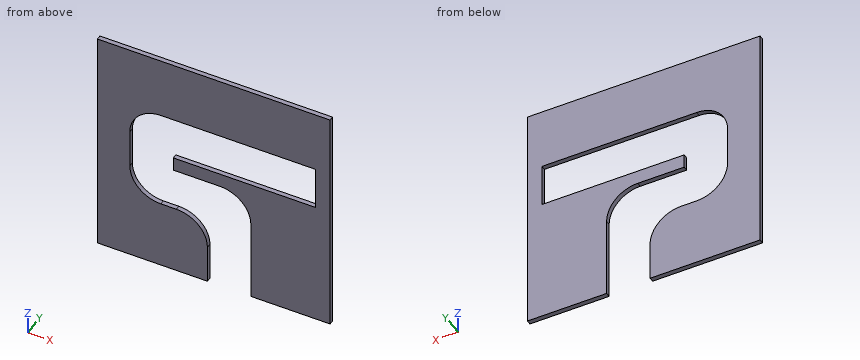
Autodesk Inventor part; units mm, degrees
ref_plane "YZ Plane" through (0, 0, 0) normal (1, 0, 0) x (0, 1, 0)
ref_plane "XZ Plane" through (0, 0, 0) normal (0, 1, 0) x (-1, 0, 0)
ref_plane "XY Plane" through (0, 0, 0) normal (0, 0, 1) x (1, 0, 0)
sketch "Esquisse1" plane through (0, 0, 0) normal (0, 1, 0) x (-1, 0, 0)
  line L0 (0, 0) -> (300, 0)
  line L1 (300, 0) -> (300, -300)
  line L2 (300, -300) -> (0, -300)
  line L3 (0, -300) -> (0, 0)
  line L4 (158.1666, -300) -> (158.1666, -290)
  line L5 (158.1666, -290) -> (158.1666, -210)
  line L6 (158.1666, -210) -> (258.1666, -210)
  line L7 (258.1666, -210) -> (258.1666, -159)
  line L8 (202.1666, -154) -> (102.1666, -154)
  line L9 (158.1666, -300) -> (102.1666, -300)
  line L10 (102.1666, -300) -> (102.1666, -154)
  line L11 (202.1666, -136) -> (102.1666, -136)
  line L12 (215.9662, -80) -> (258.1666, -80)
  line L13 (258.1666, -80) -> (258.1666, -159)
  line L14 (215.9662, -80) -> (102.1666, -80)
  line L15 (202.1666, -136) -> (202.1666, -154)
  line L16 (102.1666, -136) -> (18.7834, -136)
  line L17 (18.7834, -136) -> (18.7834, -80)
  line L18 (18.7834, -80) -> (102.1666, -80)
  dimension "d0" = 300
  dimension "d1" = 300
  dimension "d4" = 100
  dimension "d7" = 56
  dimension "d13" = 146
  dimension "d14" = 100
  dimension "d15" = 130
  dimension "d17" = 56
  dimension "d18" = 90
extrude "Extrusion2" add sketch "Esquisse1" along normal blind 6 contours L0 L1 L2 L4 L5 L6 L7 L13 L12 L14 L18 L17 L16 L11 L15 L8 L10 L3
fillet "Congé1" radius 40 4 edges at (-102.1666, 3, -154) (-158.1666, 3, -210) (-258.1666, 3, -210) (-258.1666, 3, -80)
properties part number "Plaque vois"
Model file for the job. Use its own axes, mm. Give positions to 0.01 mm unless a question says otherwise; leave off trailing zeros. Loops run counter-clockwise (first coordinate to the right, second up) from the corner with the lowest first, then second, coordinate; pieces in that order, holes last.
Item 1: Drop a flat-ended pin along its axis: P1, Ø8, axis at x = -142, z = -159, coming from the -Y side. Give the stop position or say it passes through.
Check values:
P1: passes through
Item 2: Drill centre lines: line 1 along Z through (x, y) = (-149, 1.6); line 2 along X through (y, z) = (2.25, -137.5); line 3 along X through (y, z) = (0.7, -252.5). Where is each one in solid material? Low to high.
Check values:
line 1: z = -154 to -136, -80 to 0
line 2: x = -300 to -258.17, -202.17 to 0
line 3: x = -300 to -158.17, -102.17 to 0
Item 3: Slice it at C-C (y = 1.35). Write the cut outline in (x, z), plus the area to 3 significant figures.
Check values:
outline: (-300, -300) - (-158.17, -300) - (-158.17, -250) arc R40 ccw to (-198.17, -210) - (-218.17, -210) arc R40 cw to (-258.17, -170) - (-258.17, -120) arc R40 cw to (-218.17, -80) - (-18.78, -80) - (-18.78, -136) - (-202.17, -136) - (-202.17, -154) - (-142.17, -154) arc R40 cw to (-102.17, -194) - (-102.17, -300) - (0, -300) - (0, 0) - (-300, 0) - close
area: 62,500 mm2
Item 4: Slice it at B-B (x = -85). Write the cut outline in (y, z), plus the area to 3 significant figures.
Check values:
outline: (0, -300) - (6, -300) - (6, -136) - (0, -136) - close; (0, -80) - (6, -80) - (6, 0) - (0, 0) - close
area: 1,460 mm2
Item 5: Slice it at A-A (z = -270). Write the cut outline in (x, y), plus the area to 3 significant figures.
Check values:
outline: (-300, 0) - (-158.17, 0) - (-158.17, 6) - (-300, 6) - close; (-102.17, 0) - (0, 0) - (0, 6) - (-102.17, 6) - close
area: 1,460 mm2
